The model under review builds one solid part; all positions refer to its coordinate system, in mm. A direction names the side the tool comes from. Give positions to 0.01 mm unless a question says otherwise; leave off trailing zeros. Order: outer loops, then holes, each group sorted by start corner. A loop starts at its lowest first (then second) coordinate and runs counter-clockwise, first axis right, second up. Notation, with made-up numbers: (30, 3) -> (82, 3) arc R3 cw to (82, 8) -> close; hole circle Ø7 at (70, 74.5). An arc over 180 degrees is marked (long way). Use one line per item in the form item = value.
Autodesk Inventor part; units mm, degrees
ref_plane "YZ Plane" through (0, 0, 0) normal (1, 0, 0) x (0, 1, 0)
ref_plane "XZ Plane" through (0, 0, 0) normal (0, 1, 0) x (-1, 0, 0)
ref_plane "XY Plane" through (0, 0, 0) normal (0, 0, 1) x (1, 0, 0)
sketch "Эскиз1" plane through (0, 0, 0) normal (1, 0, 0) x (0, 1, 0)
  circle A0 centre (35.2311, -22.6062) radius 9.3
  circle A1 centre (0, -38.8201) radius 6.1 construction
  circle A2 centre (0, 0) radius 4.85 construction
  circle A3 centre (35.8147, -49.5529) radius 3.55
  line L0 (6.0968, -38.6237) -> (4.8475, 0.1562) construction
  line L1 (-4.8475, 0.1562) -> (-6.0968, -38.6237) construction
  line L2 (0, 0) -> (0, -38.8201) construction
  circle A4 centre (0, -38.8201) radius 4.1
  circle A5 centre (0, 0) radius 2.5
  circle A6 centre (0, -38.8201) radius 15 construction
  circle A7 centre (0, 0) radius 14 construction
  circle A8 centre (0, -38.8201) radius 7.6
  circle A9 centre (0, 0) radius 7 construction
  line L3 (7.5465, -39.7207) -> (12.114, -1.4456)
  line L4 (-7.5465, -39.7207) -> (-12.114, -1.4456)
  circle A10 centre (0, 0) radius 8.8 construction
  circle A11 centre (0, 0) radius 12.2
  circle A12 centre (6.8983, -19.8347) radius 1.6
  circle A13 centre (-7.3019, -16.4524) radius 1.6
  point P0 (-7, 0)
  point P1 (-7.5465, -39.7207)
  point P2 (-12.114, -1.4456)
  dimension "d0" = 18.6
  dimension "d1" = 12.2
  dimension "d2" = 9.7
  dimension "d3" = 7.1
  dimension "d8" = 38.8201
  dimension "d13" = 38.8
  dimension "d14" = 38.8
  dimension "d23" = 8.2
  dimension "d24" = 5
  dimension "d25" = 30
  dimension "d26" = 28
  dimension "d28" = 14
  dimension "d31" = 17.6
  dimension "d32" = 3.4
  dimension "d56" = 3.5
  dimension "d58" = 3.2
  dimension "d59" = 3
  dimension "d60" = 21
  dimension "d61" = 3.2
  dimension "d62" = 3
  dimension "d63" = 18
extrude "Выдавливание4" add sketch "Эскиз1" along normal blind 3 contours A8 | A8 L4 A11 L3 | A11
sketch "Эскиз4" plane through (0, 0, 0) normal (-1, 0, 0) x (0, 0, 1)
  circle A0 centre (-38.8201, 0) radius 4.1 construction
  arc A1 (-1.4456, -12.114) -> (-1.4456, 12.114) centre (0, 0) ccw construction
  line L0 (-39.7207, 7.5465) -> (-1.4456, 12.114) construction
  arc A2 (-39.7207, 7.5465) -> (-39.7207, -7.5465) centre (-38.8201, 0) ccw construction
  line L1 (-1.4456, -12.114) -> (-39.7207, -7.5465) construction
  line L2 (0, 0) -> (0, 12.2) construction
  arc A3 (-1.4456, -12.114) -> (-1.4456, 12.114) centre (0, 0) ccw construction
  line L3 (0, 0) -> (12.2, 0) construction
  circle A4 centre (5.6569, 5.6569) radius 1.7
  line L4 (5.6569, 5.6569) -> (0, 0) construction
  circle A5 centre (-6.364, 6.364) radius 1.7
  line L5 (0, 0) -> (-6.364, 6.364) construction
  circle A6 centre (-5.6569, -5.6569) radius 1.7
  circle A7 centre (6.364, -6.364) radius 1.7
  dimension "d65" = 45
  dimension "d66" = 3.4
  dimension "d67" = 3.4
  dimension "d68" = 45
  dimension "d69" = 16
  dimension "d70" = 18
extrude "Выдавливание5" cut sketch "Эскиз4" against normal blind 3
sketch "Эскиз5" plane through (3, 0, 0) normal (1, 0, 0) x (0, 0, -1)
  circle A0 centre (0, 0) radius 3.75
  dimension "d38" = 7.5
extrude "Выдавливание6" cut sketch "Эскиз5" against normal blind 1
sketch "Эскиз6" plane through (3, 0, 0) normal (1, 0, 0) x (0, 0, -1)
  circle A0 centre (0, -18) radius 2
  circle A1 centre (0, 0) radius 3.75 construction
  circle A2 centre (-5.6569, 5.6569) radius 1.7 construction
  circle A3 centre (38.8201, 0) radius 4.1 construction
  line L0 (39.7207, 7.5465) -> (1.4456, 12.114) construction
  arc A4 (1.4456, 12.114) -> (1.4456, -12.114) centre (0, 0) ccw construction
  line L1 (1.4456, -12.114) -> (39.7207, -7.5465) construction
  arc A5 (39.7207, -7.5465) -> (39.7207, 7.5465) centre (38.8201, 0) ccw construction
  line L2 (0, 0) -> (0, -26.6004) construction
  circle A6 centre (0, 0) radius 14 construction
  line L3 (-10.8605, -5.5578) -> (-3.5608, -19.8222)
  arc A7 (0, -14) -> (-3.5608, -19.8222) centre (0, -18) ccw construction
  line L4 (2.8284, -20.8284) -> (12.911, -10.7458)
  line L5 (1.4456, -12.114) -> (39.7207, -7.5465) construction
  arc A8 (2.8284, -20.8284) -> (0, -14) centre (0, -18) ccw construction
  arc A9 (-3.5608, -19.8222) -> (2.8284, -20.8284) centre (0, -18) ccw
  line L6 (-10.8605, -5.5578) -> (-10.1465, -5.5578)
  line L7 (-10.1465, -5.5578) -> (-6.8136, -9.4237)
  line L8 (-6.8136, -9.4237) -> (5.1237, -10.512)
  line L9 (5.1237, -10.512) -> (12.911, -10.7458)
  dimension "d42" = 28
  dimension "d41" = 4
  dimension "d43" = 18
  dimension "d44" = 8
  dimension "d45" = 45
extrude "Выдавливание7" [suppressed]
sketch "Эскиз7" plane through (3, 0, 0) normal (1, 0, 0) x (0, 0, -1)
  line L0 (0, 0) -> (0, -29.4139) construction
  circle A0 centre (-9, -15.5885) radius 1.6
  line L1 (-9, -15.5885) -> (0, 0) construction
  circle A1 centre (0, 0) radius 14 construction
  circle A2 centre (0, 0) radius 18 construction
  arc A3 (-6.7, -19.5722) -> (-13.5823, -15.1855) centre (-9, -15.5885) ccw construction
  circle A4 centre (0, 0) radius 3.75 construction
  circle A5 centre (-5.6569, 5.6569) radius 1.7 construction
  circle A6 centre (38.8201, 0) radius 4.1 construction
  line L2 (39.7207, 7.5465) -> (1.4456, 12.114) construction
  arc A7 (1.4456, 12.114) -> (1.4456, -12.114) centre (0, 0) ccw
  line L3 (1.4456, -12.114) -> (39.7207, -7.5465)
  arc A8 (39.7207, -7.5465) -> (39.7207, 7.5465) centre (38.8201, 0) ccw construction
  line L4 (-12.1531, 1.0686) -> (-13.5823, -15.1855)
  line L5 (-6.7, -19.5722) -> (7.4613, -11.3962)
  line L6 (1.4456, -12.114) -> (39.7207, -7.5465) construction
  arc A9 (-13.5823, -15.1855) -> (-6.7, -19.5722) centre (-9, -15.5885) ccw
  circle A10 centre (-9, -15.5885) radius 4.1
  point P0 (7.4613, -11.3962)
  dimension "d48" = 3.2
  dimension "d49" = 330
  dimension "d50" = 28
  dimension "d51" = 4
  dimension "d53" = 30
  dimension "d57" = 3
  dimension "d71" = 8.2
extrude "Выдавливание8" add sketch "Эскиз7" against normal up to surface (3 mm away) contours A7 L3 L5 A9 L4 | A10
properties part number "right_wall_v1"
1. Add section D-D on z = 0. Give the boundary of the cut face in (x, y).
Values:
outline = (0, -15.7) -> (3, -15.7) -> (3, -3.75) -> (2, -3.75) -> (2, -2.5) -> (0, -2.5) -> close; (0, 2.5) -> (2, 2.5) -> (2, 3.75) -> (3, 3.75) -> (3, 12.2) -> (0, 12.2) -> close
2. Add section A-A on z = 9. Give the boundary of the cut face in (x, y).
Values:
outline = (0, -20.19) -> (3, -20.19) -> (3, -17.19) -> (0, -17.19) -> close; (0, -13.99) -> (3, -13.99) -> (3, 8.24) -> (0, 8.24) -> close
3. Add section C-C on y = 0. Give the boundary of the cut face in (x, z), then the cut area to 3 significant figures.
Values:
outline = (0, -46.42) -> (3, -46.42) -> (3, -42.92) -> (0, -42.92) -> close; (0, -34.72) -> (3, -34.72) -> (3, -3.75) -> (2, -3.75) -> (2, -2.5) -> (0, -2.5) -> close; (0, 2.5) -> (2, 2.5) -> (2, 3.75) -> (3, 3.75) -> (3, 12.25) -> (0, 12.25) -> close
area = 134 mm^2
4. The part is to be moulded in two halves that separate along Y. For faces 1 (the face through (1.48, 9.8, -20.85)), 2 (the face through (0.99, -0.54, 2.44)), 3 (the face through (1.48, 0.15, -46.42)), say which applies: +Y half, -Y half, draft (parallel to the pull), parting line (faces both ways), or undercut.
Values:
face_1 = +Y half
face_2 = undercut
face_3 = parting line
5. Tool access review of faces 4 (the face through (2, 3, 0)), 5 (the face through (3, -1, -9)): name each direction out of +Z, -Z, +X, -X, +Y, -Y from which nothing blocks a thin tool from reaching the whole face with its end or side.
Values:
face_4 = +X
face_5 = +Z, -Z, +X, +Y, -Y
6. For L1, parallel to Z at x = 1.2, y = 0; L2, parallel to Y at x = 2.9, z = 5; L3, parallel to Y at x = 2.7, z = -42.5, list the stretches that pass through material, from the lowest coordinate up.
Values:
L1 = -46.42 to -42.92, -34.72 to -2.5, 2.5 to 12.25
L2 = -18.59 to -7.38, -5.35 to 4.09, 7.22 to 11.13
L3 = -6.65 to -1.81, 1.81 to 6.65
7. Add section B-B on x = 1.1. Count the separate pieces of the cut face and the enclosed holes in it, then the cut area to 3 significant figures.
Values:
separate_pieces = 1
enclosed_holes = 9
area = 1,100 mm^2
8. For pin 1 Ø2 at (y, z) = (-6.364, 6.364) entering from -X; pin 2 Ø1.5 at (x, z) = (2.5, -24.5) entering from -Y; pin 3 Ø7 at (y, z) = (0, 0) entering from +X, all flat-tipped, find the tip position at first contact; note any pin that passes through.
Values:
pin_1 = through
pin_2 = -9.45
pin_3 = 2
